Geometry: final body of the model. Coordinates: model frame, mm. A direction names the side the tool comes from. Give positions to 0.01 mm unless a question says otherwise; leave off trailing zeros. Write each loop counter-clockwise with the first axis right and the second up, starting at its lowest first coordinate (ties: lowest second). Pieces come first, ordered by that corner, then holes. Notation, with made-up numbers: M -35,-32.5 L -27,-32.5 A24 cw -27,-21.5 Z; hole C 82.25,61 d5. An arc over 180 degrees is marked long. Use a Markdown table: item, result. Add a question column.
1) Section C-C on z = -29.5. Return the cut outline in (x, y).
2) Section A-A on z = -61.29. Return the cut outline in (x, y), then the cut area to 3 significant figures.
3) Pin query (flat end, axial travel): pin 1 (2.5 mm diameter, centred on x = 1.5, y = -3, fed in from +Z); pin 2 (1 mm diameter, centred on x = 55.5, z = -69, fed in from -Y); pin 3 (1.9 mm diameter, centred on x = 67.06, z = -67.29, fed in from +Y); pin 4 (1.5 mm diameter, centred on x = 1.5, y = -2.5, fed in from -Z). Return the tip coordinate at first contact, or that it passes through.
4) Set-up query: faces 5 (the flat face through (3, -4, -30)), 6 (the flat face through (1, -4, -12.1)), 7 (the flat face through (1, -4, -47.1)), 8 (the flat face through (0, 1, -51)). Return all of +Z, -Z, +X, -X, +Y, -Y with unobstructed straight access to the full face (end or side cutting, diameter ignored); none if empty.
5) Line query: line 1 (Y direction, x = 20.5, z = -95); line 2 (X direction, y = 1.35, z = -61.29). Output: solid intervals per line, ascending.
6) Section D-D on x = 12. Return the cut outline in (y, z), then the cut area to 3 significant figures.
7) Draft query along Y for faces 1 (the cylindrical face through (1.48, -3.17, -34.59)), 2 (the flat face through (1, -9, -29)), 3 (the cylindrical face through (1.48, -3.44, -24.93)), 4 (the flat face through (37, 3, -66)). Return one class per face: +Y half, -Y half, draft (parallel to the pull), parting line (faces both ways), or undercut.
8) Section B-B on y = -4.5. Return the cut outline in (x, z).
```python
from build123d import *

# Parameters (mm, degrees)
SKETCH1_W           = 134.58
SKETCH1_H           = 3
BOSS_EXTRUDE1_DEPTH = 75
SKETCH2_W           = 3
SKETCH2_H           = 35
BOSS_EXTRUDE2_DEPTH = 9
SKETCH3_R           = 1.575
CUT_EXTRUDE1_DEPTH  = 155.330089095
SKETCH5_R           = 1.575
CUT_EXTRUDE2_DEPTH  = 155.534062265


with BuildPart() as part:
    # Sketch1 → Boss-Extrude1 (new body)
    with BuildSketch(Plane(origin=(0, 0, 0), x_dir=(0, 0, -1), z_dir=(1, 0, 0))):
        with Locations((67.29, 1.5)):
            Rectangle(SKETCH1_W, SKETCH1_H)
    extrude(amount=BOSS_EXTRUDE1_DEPTH)

    # Sketch2 → Boss-Extrude2 (add)
    with BuildSketch(Plane.XZ):
        with Locations((1.5, -29.6)):
            Rectangle(SKETCH2_W, SKETCH2_H)
    extrude(amount=BOSS_EXTRUDE2_DEPTH)

    # Sketch3 → Cut-Extrude1 (cut, through all)
    with BuildSketch(Plane.ZY):
        with Locations((-23.766666667, -4.5)):
            Circle(SKETCH3_R)
        with Locations((-35.433333333, -4.5)):
            Circle(SKETCH3_R)
    extrude(amount=-CUT_EXTRUDE1_DEPTH, mode=Mode.SUBTRACT)

    # Sketch5 → Cut-Extrude2 (cut, through all)
    with BuildSketch(Plane(origin=(0, 3, 0), x_dir=(1, 0, 0), z_dir=(0, 1, 0))):
        with Locations(Location((67.059177496, 61.29, 0), (0, 0, 270))):
            Circle(SKETCH5_R)
        with Locations(Location((67.059177496, 67.29, 0), (0, 0, 270))):
            Circle(SKETCH5_R)
    extrude(amount=-CUT_EXTRUDE2_DEPTH, mode=Mode.SUBTRACT)


solid = part.part
```
Found:
| question | item | result |
|---|---|---|
| 1 | outline | M 0,-9 L 3,-9 L 3,0 L 75,0 L 75,3 L 0,3 Z |
| 2 | outline | M 0,0 L 65.48,0 L 65.48,3 L 0,3 Z; M 68.63,0 L 75,0 L 75,3 L 68.63,3 Z |
| 2 | area | 216 mm² |
| 3 | pin 1 | z = -12.1 |
| 3 | pin 2 | y = 0 |
| 3 | pin 3 | through |
| 3 | pin 4 | z = -47.1 |
| 4 | face 5 | +Z, -Z, +X, -Y |
| 4 | face 6 | +Z, +X, -X, -Y |
| 4 | face 7 | -Z, +X, -X, -Y |
| 4 | face 8 | +Z, -Z, -X, +Y, -Y |
| 5 | line 1 | 0 to 3 |
| 5 | line 2 | 0 to 65.48, 68.63 to 75 |
| 6 | outline | M 0,-134.58 L 3,-134.58 L 3,0 L 0,0 Z |
| 6 | area | 404 mm² |
| 7 | face 1 | undercut |
| 7 | face 2 | -Y half |
| 7 | face 3 | undercut |
| 7 | face 4 | +Y half |
| 8 | outline | M 0,-47.1 L 3,-47.1 L 3,-37.01 L 0,-37.01 Z; M 0,-33.86 L 3,-33.86 L 3,-25.34 L 0,-25.34 Z; M 0,-22.19 L 3,-22.19 L 3,-12.1 L 0,-12.1 Z |
